```python
from build123d import *

# Parameters (mm, degrees)
F1_DEPTH  = 3.6
F2_SIZE2  = 3.59999
F2_SIZE   = 3.59999
F3_R      = 1.8
F4_R      = 1.79999
F5_R      = 1.8
F6_R      = 1.79999
F7_R      = 1.8
F8_R      = 1.79999
F9_R      = 1.1
F10_DEPTH = 2.5
F11_R     = 1.1
F12_DEPTH = 2.5


# Not quite as in the source:
# - a fillet or chamfer is up to 0.001 mm smaller than in the source, because OpenCascade refuses the exact size


with BuildPart() as f1:
    # F0 (on Top) → F1 (new body)
    with BuildSketch(Plane.XY):
        Polygon((24.4, 0), (0, 0), (0, -2.1), (9.3, -2.1), (9.3, -4.375), (0, -4.375), (0, -10.125), (9.3, -10.125), (9.3, -12.4), (0, -12.4), (0, -14.5), (22.6, -14.5), align=None)
    extrude(amount=F1_DEPTH)

    # F2 (size 3.6 and 3.6 in the source; OpenCascade refuses exactly that, so slightly less here)
    f2_edges = [f1.edges().sort_by_distance(p)[0] for p in [
        (23.5, -7.25, 3.6),
    ]]
    chamfer(f2_edges, length=F2_SIZE, length2=F2_SIZE2)

    # F3
    f3_edges = [f1.edges().sort_by_distance(p)[0] for p in [
        (0, -7.25, 3.6),
    ]]
    fillet(f3_edges, radius=F3_R)

    # F4 (radius 1.8 in the source; OpenCascade refuses exactly that, so slightly less here)
    f4_edges = [f1.edges().sort_by_distance(p)[0] for p in [
        (0, -7.25, 0),
    ]]
    fillet(f4_edges, radius=F4_R)

    # F5
    f5_edges = [f1.edges().sort_by_distance(p)[0] for p in [
        (0, -13.45, 3.6),
    ]]
    fillet(f5_edges, radius=F5_R)

    # F6 (radius 1.8 in the source; OpenCascade refuses exactly that, so slightly less here)
    f6_edges = [f1.edges().sort_by_distance(p)[0] for p in [
        (0, -13.45, 0),
    ]]
    fillet(f6_edges, radius=F6_R)

    # F7
    f7_edges = [f1.edges().sort_by_distance(p)[0] for p in [
        (0, -1.05, 3.6),
    ]]
    fillet(f7_edges, radius=F7_R)

    # F8 (radius 1.8 in the source; OpenCascade refuses exactly that, so slightly less here)
    f8_edges = [f1.edges().sort_by_distance(p)[0] for p in [
        (0, -1.05, 0),
    ]]
    fillet(f8_edges, radius=F8_R)

    # F9 (on face) → F10 (join)
    with BuildSketch(Plane.XZ.offset(14.5)):
        with Locations((1.8, 1.8)):
            Circle(F9_R)
    extrude(amount=F10_DEPTH)

    # F11 (on face) → F12 (join)
    with BuildSketch(Plane(origin=(0, 0, 0), x_dir=(-1, 0, 0), z_dir=(0, 1, 0))):
        with Locations((-1.8, 1.8)):
            Circle(F11_R)
    extrude(amount=F12_DEPTH)


solid = f1.part
```
Model file for the job. Use its own axes, mm. A direction names the side the tool comes from. Coordinates: 2 decimals unless noted, no trailing zeros. Write each loop counter-clockwise with the first axis right and the second up, starting at its lowest first coordinate (ties: lowest second). Pieces come first, ordered by that corner, then holes. Notation, with made-up numbers: (28, -15.75) - (54, -15.75) arc R27 ccw to (54, 20.25) - close; hole circle Ø10 at (53.5, 49). An arc over 180 degrees is marked (long way). One line per question, with ' | ' between items. Start each with the question number.
Q1. Cut at D-D, the plane x = 10. List the corners of the cut face in (y, z), then the cut area to 3 significant figures.
Q2. Pin check, flat tips, straight feed: pin 1 (2 mm diameter, centred on x = 9.5, z = 2.5, fed in from +Y); pin 2 (2 mm diameter, centred on x = 12, z = 1, fed in from -Y); pin 3 (2 mm diameter, centred on y = -15, z = 2, fed in from +X). Stop position of each tip, or through.
Q3. Pull direction Y, two halves, no side cores. Call faces 4 (the face through (9.3, -11, 2)), 5 (the face through (21.648, -7.351, 1.825)), 6 (the face through (0.989, -15.732, 2.543)): pulls with the +Y half, pulls with the -Y half, needs draft (parallel to the pull), parting line crosses it, or undercut.
Q4. Cut at B-B, the plane z = 1.35. List the corners of the cut face in (x, y) (3 decimals), then the cut area to 3 significant figures.
Q5. Drill centre lines: line 1 (Y direction, x = 6.25, z = 1.85) (3 decimals); line 2 (Y direction, x = 16.25, z = 3.05); line 3 (X direction, y = -10.75, z = 2.45). Where is each one in solid material? Low to high. Write a range as [from, to].
Q6. Cut at A-A, the plane x = 5.75. List the corners of the cut face in (y, z) (3 decimals), then the cut area to 3 significant figures.
Q7. 3-axis set-ups, long thin cutter, end or side, ignore diameter. For faces 1 (the face through (5, -2.1, 2)), 2 (the face through (2.611, 1.232, 2.543)), 3 (the face through (0.513, -1.065, 0.541)): which of +Z, -Z, +X, -X, +Y, -Y reach the whole face in a straight line?
Answer below:
1) outline: (-14.5, 0) - (0, 0) - (0, 3.6) - (-14.5, 3.6) - close | area: 52.2 mm^2
2) pin 1: y = 0 | pin 2: y = -14.5 | pin 3: x = 21.46
3) face 4: undercut | face 5: pulls with the -Y half | face 6: needs draft
4) outline: (0.057, -14.5) - (0.796, -14.5) - (0.796, -17) - (2.804, -17) - (2.804, -14.5) - (21.24, -14.5) - (23.04, 0) - (2.804, 0) - (2.804, 2.5) - (0.796, 2.5) - (0.796, 0) - (0.057, 0) - (0.057, -2.1) - (9.3, -2.1) - (9.3, -4.375) - (0.057, -4.375) - (0.057, -10.125) - (9.3, -10.125) - (9.3, -12.4) - (0.057, -12.4) - close | area: 288 mm^2
5) line 1: [-14.5, -12.4], [-10.125, -4.375], [-2.1, 0] | line 2: [-14.5, 0] | line 3: [9.3, 20.6]
6) outline: (-14.5, 0) - (-12.4, 0) - (-12.4, 3.6) - (-14.5, 3.6) - close; (-10.125, 0) - (-4.375, 0) - (-4.375, 3.6) - (-10.125, 3.6) - close; (-2.1, 0) - (0, 0) - (0, 3.6) - (-2.1, 3.6) - close | area: 35.8 mm^2
7) face 1: +Z, -Z, -X | face 2: +Y | face 3: -Z, -X, +Y, -Y
